```python
from build123d import *

# Parameters (mm, degrees)
CBORE_FOR_00_BINDING_HEAD_MACHINE_S_2_COUNT = 2
CBORE_FOR_00_BINDING_HEAD_MACHINE_S_2_PITCH = 6.363961031
CBORE_FOR_00_BINDING_HEAD_MACHINE_S_3_COUNT = 2
CBORE_FOR_00_BINDING_HEAD_MACHINE_S_3_PITCH = 9
CBORE_FOR_00_BINDING_HEAD_MACHINE_S_4_COUNT = 2
CBORE_FOR_00_BINDING_HEAD_MACHINE_S_4_PITCH = 6.363961031
SKETCH10_R                                  = 1.2
CUT_EXTRUDE1_DEPTH                          = 20.386059671
SKETCH11_R                                  = 1.266741203
CUT_EXTRUDE2_DEPTH                          = 4


with BuildPart() as part:
    # Sketch1 → Revolve1 (revolve)
    with BuildSketch(Plane.XY, mode=Mode.PRIVATE) as revolve1_sk:
        Polygon((-5.813736264, 6.85), (-5.813736264, -7.65), (2.186263736, -7.65), (2.186263736, -4.15), (-3.813736264, -4.15), (-3.813736264, 6.85), align=None)
    revolve(revolve1_sk.sketch.rotate(Axis((-5.813736264, 6.85, 0), (0, -1, 0)), 180), axis=Axis((-5.813736264, 6.85, 0), (0, -1, 0)))

    # Sketch7 → CBORE for #00 Binding Head Machine Screw1 (revolve, cut)
    with BuildSketch(Plane(origin=(-10.313736264, -4.15, 0), x_dir=(0, 0, 1), z_dir=(1, 0, 0))):
        Polygon((0, 0), (0, 0.469701142), (0.6985, 0.05), (0.6985, 0.7112), (1.5875, 0.7112), (1.5875, 0.635), (2.2225, 0), align=None)
    cbore_for_00_binding_head_machine_screw = revolve(axis=Axis((-10.313736264, 2.2, 0), (0, -1, 0)), mode=Mode.SUBTRACT)

    # CBORE for _00 Binding Head Machine S 2: CBORE for #00 Binding Head Machine Screw1 ×2
    with Locations(*[Vector(0.7071067811865475, 0, -0.7071067811865477) * (i * CBORE_FOR_00_BINDING_HEAD_MACHINE_S_2_PITCH) for i in range(1, CBORE_FOR_00_BINDING_HEAD_MACHINE_S_2_COUNT)]):
        add(cbore_for_00_binding_head_machine_screw, mode=Mode.SUBTRACT)

    # CBORE for _00 Binding Head Machine S 3: CBORE for #00 Binding Head Machine Screw1 ×2
    with Locations(*[(i * CBORE_FOR_00_BINDING_HEAD_MACHINE_S_3_PITCH, 0, 0) for i in range(1, CBORE_FOR_00_BINDING_HEAD_MACHINE_S_3_COUNT)]):
        add(cbore_for_00_binding_head_machine_screw, mode=Mode.SUBTRACT)

    # CBORE for _00 Binding Head Machine S 4: CBORE for #00 Binding Head Machine Screw1 ×2
    with Locations(*[Vector(0.7071067811865475, 0, 0.7071067811865477) * (i * CBORE_FOR_00_BINDING_HEAD_MACHINE_S_4_PITCH) for i in range(1, CBORE_FOR_00_BINDING_HEAD_MACHINE_S_4_COUNT)]):
        add(cbore_for_00_binding_head_machine_screw, mode=Mode.SUBTRACT)

    # Sketch10 → Cut-Extrude1 (cut, through all)
    with BuildSketch(Plane(origin=(0, -4.15, 0), x_dir=(1, 0, 0), z_dir=(0, 1, 0))):
        with Locations(Location((-10.313736264, 0, 0), (0, 0, 180))):
            Circle(SKETCH10_R)
        with Locations(Location((-5.813736264, 4.5, 0), (0, 0, 180))):
            Circle(SKETCH10_R)
        with Locations(Location((-1.313736264, 0, 0), (0, 0, 180))):
            Circle(SKETCH10_R)
        with Locations(Location((-5.813736264, -4.5, 0), (0, 0, 180))):
            Circle(SKETCH10_R)
    extrude(amount=-CUT_EXTRUDE1_DEPTH, mode=Mode.SUBTRACT)

    # Sketch11 → Cut-Extrude2 (cut)
    with BuildSketch(Plane.XZ.offset(7.65)):
        with Locations((-5.813736264, 0)):
            Circle(SKETCH11_R)
    extrude(amount=-CUT_EXTRUDE2_DEPTH, mode=Mode.SUBTRACT)


solid = part.part
```
Input: part model. Units: mm. Frame: model coordinates. A direction names the side the tool comes from. Coordinates: 2 decimals unless noted, no trailing zeros. Loops run counter-clockwise (first coordinate to the right, second up) from the corner with the lowest first, then second, coordinate; pieces in that order, holes last. Notation, with made-up numbers: M -22.5,21 L 28.5,21 A25 cw 28.5,37 Z; hole C 57.25,28 d2. An arc over 180 degrees is marked long. Answer in a Markdown table with one row per item.
1. Section B-B, the plane y = -5.75. Output: boundary loops of the cut face in (x, z), then the cut area to 3 significant figures.
Response:
| item | result |
|---|---|
| outline | C -5.81,0 d16; hole C -10.31,0 d2.4; hole C -5.81,0 d2.53; hole C -5.81,-4.5 d2.4; hole C -5.81,4.5 d2.4; hole C -1.31,0 d2.4 |
| area | 178 mm2 |
2. Section D-D, the plane y = 4.5. Output: boundary loops of the cut face in (x, z), then the cut area to 3 significant figures.
Response:
| item | result |
|---|---|
| outline | C -5.81,0 d4 |
| area | 12.6 mm2 |
3. Reachability of faces 4 (the cylindrical face through (-13.204, -5.876, 3.064)), 5 (the flat face through (-6, -3.65, 0)) from +Z, -Z, +X, -X, +Y, -Y: full face, straight path, thin tool, end or side. Return the list, or none.
Response:
| item | result |
|---|---|
| face 4 | +Y, -Y |
| face 5 | -Y |
4. Material intervals for line 1 (Y direction, x = -0.25, z = 5); line 2 (Z direction, x = -12, y = -4.25); line 3 (X direction, y = -4.75, z = 4.5), sorted ascending.
Response:
| item | result |
|---|---|
| line 1 | y = -7.65 to -4.15 |
| line 2 | z = -5.07 to -1.29, 1.29 to 5.07 |
| line 3 | x = -12.43 to -7.44, -4.19 to 0.8 |
5. Section C-C, the plane z = 4.5. Output: boundary loops of the cut face in (x, y) (3 decimals).
Response:
| item | result |
|---|---|
| outline | M -12.428,-7.65 L -7.014,-7.65 L -7.014,-4.861 L -7.401,-4.861 L -7.401,-4.785 L -8.036,-4.15 L -12.428,-4.15 Z; M -4.614,-7.65 L 0.801,-7.65 L 0.801,-4.15 L -3.591,-4.15 L -4.226,-4.785 L -4.226,-4.861 L -4.614,-4.861 Z |
6. Section A-A, the plane z = 0. Count the separate pieces of the cut face and the enclosed holes in it, then the cut area to 3 significant figures.
Response:
| item | result |
|---|---|
| separate pieces | 3 |
| enclosed holes | 0 |
| area | 71.2 mm2 |
7. Draft query along Z for faces 1 (the cylindrical face through (-4.23, 1.43, 1.22)), 2 (the flat face through (-7, -4.15, 2)), 3 (the cylindrical face through (-0.115, -6.236, 0.053)). Return one class per face: pulls with the +Z half, pulls with the -Z half, needs draft (parallel to the pull), parting line crosses it, or undercut.
Response:
| item | result |
|---|---|
| face 1 | parting line crosses it |
| face 2 | needs draft |
| face 3 | undercut |
8. First-contact query: pin 1 (2 mm diameter, centred on y = 1.5, z = 2, fed in from -X); pin 2 (4 mm diameter, centred on x = -8.5, y = 3, fed in from -Z); pin 3 (2.5 mm diameter, centred on x = -2, z = -0.5, fed in from +Y). Flat tips, straight axial feed; report the tip coordinate or a pass-through.
Response:
| item | result |
|---|---|
| pin 1 | stops at x = -7.55 |
| pin 2 | stops at z = -1.88 |
| pin 3 | stops at y = -4.27 |
